Can you work these out from the model? Positions are in its coordinate system, mm. Give positions to 0.01 mm unless a question says otherwise; leave off trailing zeros. Write each loop counter-clockwise with the first axis right and the second up, starting at its lowest first coordinate (ties: lowest second). Pieces come first, ordered by that corner, then holes.
```python
from build123d import *

# Parameters (mm, degrees)
SKETCH1_W           = 127.635
SKETCH1_H           = 127.635
MAIN_PLATE_DEPTH    = 12.7
SKETCH9_R           = 85.725
BOSS_EXTRUDE1_DEPTH = 12.7
SKETCH10_R          = 97.039626961
SKETCH10_R_2        = 83.82
CUT_EXTRUDE1_DEPTH  = 167.64


with BuildPart() as part:
    # Sketch1 → Main Plate (new body)
    with BuildSketch(Plane(origin=(0, 0, 0), x_dir=(1, 0, 0), z_dir=(0, 1, 0))):
        with Locations((63.8175, 63.8175)):
            Rectangle(SKETCH1_W, SKETCH1_H)
    extrude(amount=MAIN_PLATE_DEPTH)

    # Sketch9 → Boss-Extrude1 (add)
    with BuildSketch(Plane(origin=(0, 12.7, 0), x_dir=(1, 0, 0), z_dir=(0, 1, 0))):
        with Locations((63.8175, 63.8175)):
            Circle(SKETCH9_R)
    extrude(amount=-BOSS_EXTRUDE1_DEPTH)

    # Sketch10 → Cut-Extrude1 (cut)
    with BuildSketch(Plane(origin=(0, 12.7, 0), x_dir=(1, 0, 0), z_dir=(0, 1, 0))):
        with Locations((63.8175, 63.8175)):
            Circle(SKETCH10_R)
        with Locations(Location((63.8175, 63.8175, 0), (0, 0, 270))):
            Circle(SKETCH10_R_2, mode=Mode.SUBTRACT)
    extrude(amount=-CUT_EXTRUDE1_DEPTH, mode=Mode.SUBTRACT)


solid = part.part
```
1) Please list where these lines run through material, in increasing order: L1, parallel to X at y = 10.5, z = -64.5; L2, parallel to X at y = 6.5, z = -111; L3, parallel to Z at x = 12, y = 1.5.
Values follow:
L1: x = -20 to 147.63
L2: x = -5.46 to 133.1
L3: z = -129.7 to 2.07
2) Suppose I cut it at C-C on y = 8. Write out the boundary of the cut face in (x, z).
Values follow:
outline: circle Ø167.64 at (63.82, -63.82)
3) For pin 1 Ø3 at (y, z) = (3.5, -108) entering from -X; pin 2 Ø1.5 at (x, y) = (54, 5) entering from -Z; pin 3 Ø1.5 at (x, y) = (36.5, 1.5) entering from -Z; pin 4 Ø4 at (x, z) = (31, -48) entering from -Y, each with a flat end and sliding along its axis, tell me the tip position at first contact or that it passes through.
Values follow:
pin 1: stops at x = -8.32
pin 2: stops at z = -147.15
pin 3: stops at z = -143.32
pin 4: stops at y = 0
4) Suppose I cut it at A-A on x = 46.5. Write out the boundary of the cut face in (y, z).
Values follow:
outline: (0, -145.83) - (12.7, -145.83) - (12.7, 18.19) - (0, 18.19) - close
5) Suppose I cut it at B-B on z = -15.5. Write out the boundary of the cut face in (x, y), plus the area to 3 significant figures.
Values follow:
outline: (-4.67, 0) - (132.31, 0) - (132.31, 12.7) - (-4.67, 12.7) - close
area: 1,740 mm2
